Verification items for the finished model (mm, model axes). A direction names the side the tool comes from. Coordinates: 2 decimals unless noted, no trailing zeros. Write each loop counter-clockwise with the first axis right and the second up, starting at its lowest first coordinate (ties: lowest second). Pieces come first, ordered by that corner, then holes. Notation, with made-up numbers: (-31.5, 18) -> (-14.5, 18) arc R32 cw to (-14.5, 48) -> close; hole circle Ø5 at (37, -25.5). An arc over 180 degrees is marked (long way). Write each question's results on one line, items separated by ' | '. Start each with the question number.
from build123d import *

# Parameters (mm, degrees)
CUT_EXTRUDE1_START = 27.5
CUT_EXTRUDE1_DEPTH = 10
CUT_EXTRUDE2_START = 36
CUT_EXTRUDE2_DEPTH = 10
CHAMFER1_SIZE      = 1.5
CHAMFER2_SIZE      = 1


with BuildPart() as part:
    # Sketch1 → Revolve1 (revolve)
    with BuildSketch(Plane(origin=(0, 0, 0), x_dir=(0, 0, -1), z_dir=(1, 0, 0))):
        Polygon((0, 0), (0, 35), (140, 35), (140, 40), (224, 40), (224, 45), (412, 45), (412, 30), (470, 30), (470, 0), align=None)
    revolve(axis=Axis((0, 0, -470), (0, 0, 1)))

    # Sketch2 → Cut-Extrude1 (cut)
    with BuildSketch(Plane(origin=(0, 0, 0), x_dir=(1, 0, 0), z_dir=(0, 1, 0)).offset(CUT_EXTRUDE1_START)):
        with BuildLine():
            Line((-10, 15), (-10, 115))
            ThreePointArc((-10, 115), (0, 125), (10, 115))
            Line((10, 115), (10, 15))
            ThreePointArc((10, 15), (0, 5), (-10, 15))
        make_face()
    extrude(amount=CUT_EXTRUDE1_DEPTH, mode=Mode.SUBTRACT)

    # Sketch4 → Cut-Extrude2 (cut)
    with BuildSketch(Plane(origin=(0, 0, 0), x_dir=(1, 0, 0), z_dir=(0, 1, 0)).offset(CUT_EXTRUDE2_START)):
        with BuildLine():
            Line((12.5, 387), (12.5, 287))
            ThreePointArc((12.5, 287), (0, 274.5), (-12.5, 287))
            Line((-12.5, 287), (-12.5, 387))
            ThreePointArc((-12.5, 387), (0, 399.5), (12.5, 387))
        make_face()
    extrude(amount=CUT_EXTRUDE2_DEPTH, mode=Mode.SUBTRACT)

    # Chamfer1
    chamfer1_edges = [part.edges().sort_by_distance(p)[0] for p in [
        (0, -35, 0),
        (0, -30, -470),
    ]]
    chamfer(chamfer1_edges, length=CHAMFER1_SIZE)

    # Chamfer2
    chamfer2_edges = [part.edges().sort_by_distance(p)[0] for p in [
        (0, -40, -140),
        (0, -45, -412),
        (0, -45, -224),
    ]]
    chamfer(chamfer2_edges, length=CHAMFER2_SIZE)


solid = part.part
1. Depth check by flat-ended pin: pin 1 Ø4 at (x, z) = (27, -272.5) entering from -Y; pin 2 Ø2 at (y, z) = (41.5, -353) entering from -X; pin 3 Ø1.5 at (y, z) = (31.5, -287) entering from +X. Enter the tip coordinate at first touch or a pass-through.
2. Mould release check, pull along X, two halves, no side actions. Record for faces 4 (the cylindrical face through (39.923, 20.765, -319.302)), 5 (the flat face through (9, 29, -412)), 6 (the flat face through (0, 27.5, -66)): +X half, -X half, draft (parallel to the pull), parting line (faces both ways), or undercut.
3. Sectioned sample at C-C on z = -183. Record the cut outline in (x, y).
4. Sectioned sample at B-B on z = -292. Record the cut outline in (x, y), plus the area to 3 significant figures.
5. Tool access check on faces 1 (the flat face through (0, 0, 0)), 2 (the cylindrical face through (0.275, 40.437, -274.503)), 3 (the flat face through (39, -10, -224)). Record the directions out of +Z, -Z, +X, -X, +Y, -Y that give a thin tool (end or side, any length) a straight path to the whole face; none if there is none.
6. Material ranges on probe 1 along X at (y, z) = (-30, -311.5); probe 2 along X at (y, z) = (32, -92); probe 3 along Z at (x, y) = (25, -36), recorded low to high. Write a range as from..to.
Computed values:
1) pin 1: stops at y = -37.42 | pin 2: stops at x = -19.62 | pin 3: stops at x = 32.85
2) face 4: parting line | face 5: draft | face 6: undercut
3) outline: circle Ø80 at (0, 0)
4) outline: (-12.5, 36) -> (-12.5, 43.23) arc R45 ccw (long way) to (12.5, 43.23) -> (12.5, 36) -> close | area: 6,150 mm^2
5) face 1: +Z, +X, -X, +Y, -Y | face 2: +Y | face 3: +Z
6) probe 1: x = -33.54..33.54 | probe 2: x = -14.18..-10, 10..14.18 | probe 3: z = -412..-224
